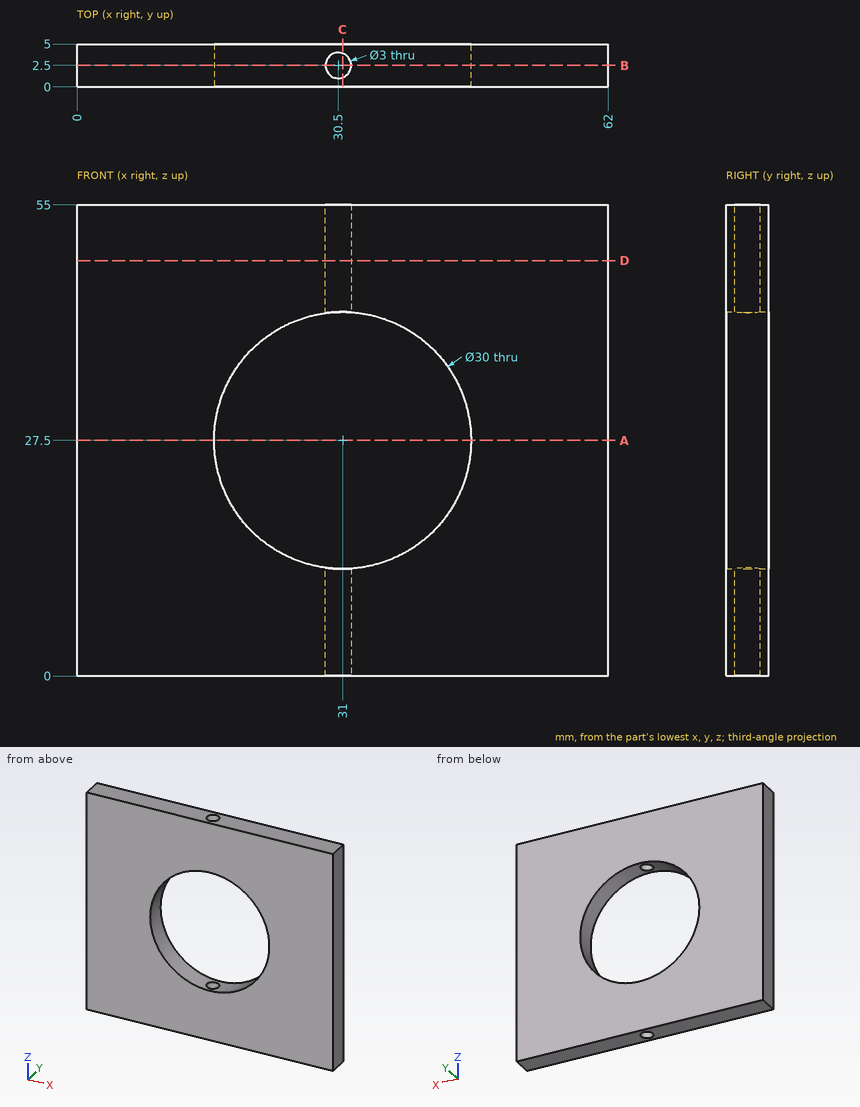
Study the drawing (mm; zero at the part's minimum x, y, z) and answer. Give positions to 0.01 mm unless a question says otherwise; leave off trailing zeros. Loops run counter-clockwise (first coordinate to the right, second up) from the corner with the lowest first, then second, coordinate; pieces in that order, holes last. Notation, with made-up numbers: (54, 80.25) - (113, 80.25) arc R24 cw to (113, 105.25) - close; hole circle Ø10 at (-10, 38). An arc over 180 degrees is marked (long way). Return JSON: item names as keys, results as strings. Group by question number.
1. Find section D-D (z = 48.5). Write down the section's boundary in (x, y), then the cut area to 3 significant figures.
2. Find section C-C (x = 31). Write down the section's boundary in (y, z), then the cut area to 3 significant figures.
3. Given pin 1 Ø2.5 at (x, y) = (30.5, 2.5) entering from +Z, flat-ended and moving along its own axis, determine where the tip first touches the part or whether it passes through.
4. Find section A-A (z = 27.5). Write down the section's boundary in (x, y), then the cut area to 3 significant figures.
5. Straight lines are drawn through the part: line 1 (Y direction, x = 30.5, z = 5); line 2 (Z direction, x = 31, y = 4); line 3 (X direction, y = 2.65, z = 9.5). For each, find the intervals that lie inside material, in ascending order. Write a range as [from, to].
6. Find section B-B (y = 2.5). Write down the section's boundary in (x, z), then the cut area to 3 significant figures.
Verdict:
{
 "1": {"outline": "(0, 0) - (62, 0) - (62, 5) - (0, 5) - close; hole circle Ø3 at (30.5, 2.5)", "area": "303 mm^2"},
 "2": {"outline": "(0, 0) - (1.09, 0) - (1.09, 12.5) - (0, 12.5) - close; (0, 42.5) - (1.09, 42.5) - (1.09, 55) - (0, 55) - close; (3.91, 0) - (5, 0) - (5, 12.5) - (3.91, 12.5) - close; (3.91, 42.5) - (5, 42.5) - (5, 55) - (3.91, 55) - close", "area": "54.3 mm^2"},
 "3": {"pin 1": "passes through"},
 "4": {"outline": "(0, 0) - (16, 0) - (16, 5) - (0, 5) - close; (46, 0) - (62, 0) - (62, 5) - (46, 5) - close", "area": "160 mm^2"},
 "5": {"line 1": "y = [0, 1], [4, 5]", "line 2": "z = [0, 12.5], [42.5, 55]", "line 3": "x = [0, 29.01], [31.99, 62]"},
 "6": {"outline": "(0, 0) - (29, 0) - (29, 12.63) arc R15 cw to (29, 42.37) - (29, 55) - (0, 55) - close; (32, 0) - (62, 0) - (62, 55) - (32, 55) - (32, 42.47) arc R15 cw to (32, 12.53) - close", "area": "2,630 mm^2"}
}
